Geometry check sheet. Reference: drawing and pictorial views, mm from the part's lowest x, y, z. Give positions to 0.01 mm unless a question says otherwise; leave off trailing zeros. Order: outer loops, then holes, each group sorted by start corner. A loop starts at its lowest first (then second) coordinate and runs counter-clockwise, first axis right, second up.
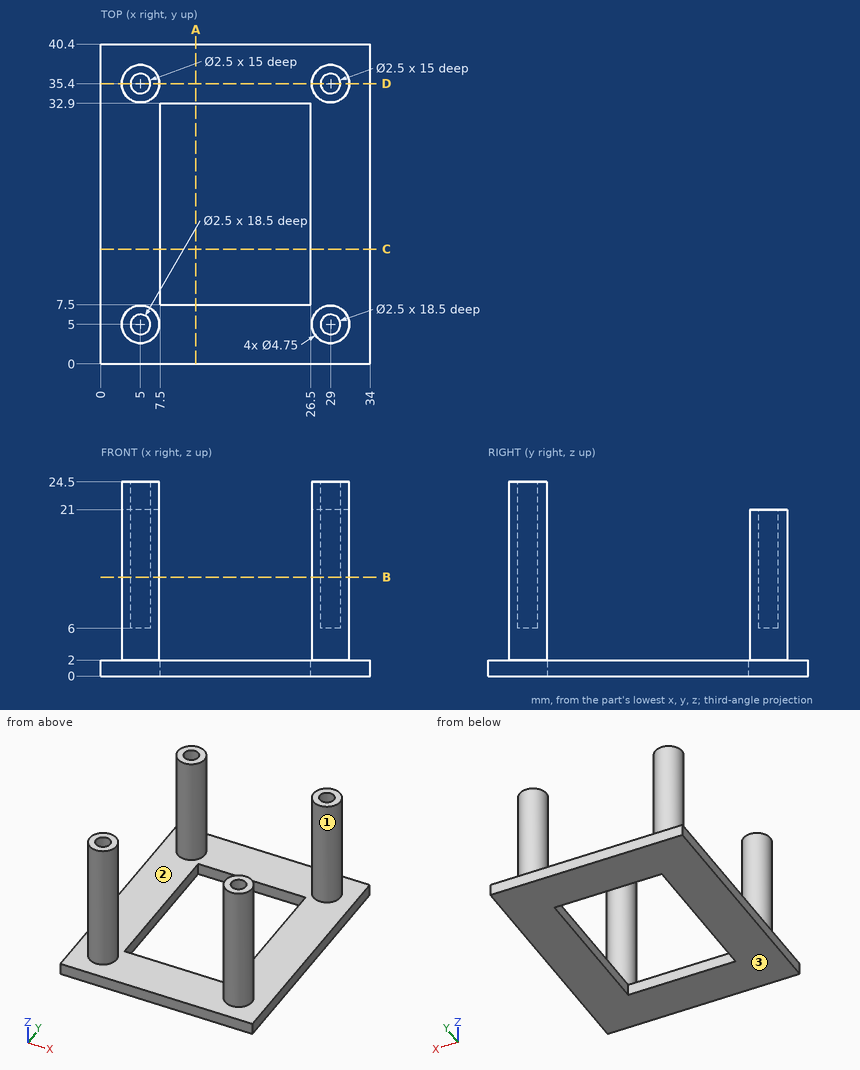
1) Depth check by flat-ended pin: pin 1 Ø1.5 at (x, y) = (5, 5) entering from +Z; pin 2 Ø4 at (x, z) = (8.5, 6.5) entering from -Y; pin 3 Ø1.6 at (x, z) = (16.5, 0.5) entering from -Y; pin 4 Ø3 at (x, y) = (4.5, 35.5) entering from +Z. Enter the tip coordinate at first touch or a pass-through.
Recorded:
pin 1: stops at z = 6
pin 2: stops at y = 3.16
pin 3: stops at y = 0
pin 4: stops at z = 21
2) Section check D-D, the plane y = 35.4. Record the cut outline in (x, z) (3 decimals).
Recorded:
outline: (0, 0) - (34, 0) - (34, 2) - (31.375, 2) - (31.375, 21) - (30.25, 21) - (30.25, 6) - (27.75, 6) - (27.75, 21) - (26.625, 21) - (26.625, 2) - (7.375, 2) - (7.375, 21) - (6.25, 21) - (6.25, 6) - (3.75, 6) - (3.75, 21) - (2.625, 21) - (2.625, 2) - (0, 2) - close
3) Material ranges on L1, parallel to Y at x = 29, z = 11.5 (3 decimals); L2, parallel to Z at x = 27, y = 25; L3, parallel to Y at x = 3, z = 3.25, recorded low to high.
Recorded:
L1: y = 2.625 to 3.75, 6.25 to 7.375, 33.025 to 34.15, 36.65 to 37.775
L2: z = 0 to 2
L3: y = 3.72 to 6.28, 34.12 to 36.68
4) Section check B-B, the plane z = 12.5. Record the cut outline in (x, y) (3 decimals), then the cut area to 3 significant figures.
Recorded:
outline: circle Ø4.75 at (5, 5); circle Ø4.75 at (5, 35.4); circle Ø4.75 at (29, 5); circle Ø4.75 at (29, 35.4); hole circle Ø2.5 at (5, 5); hole circle Ø2.5 at (5, 35.4); hole circle Ø2.5 at (29, 5); hole circle Ø2.5 at (29, 35.4)
area: 51.2 mm2
5) Draft check along Y on the marked faces 1, 2 and 3. Enter one of: +Y half, -Y half, draft (parallel to the pull), parting line (faces both ways), or undercut.
Recorded:
face 1: undercut
face 2: undercut
face 3: draft
6) Section check C-C, the plane y = 14.5. Record the cut outline in (x, z).
Recorded:
outline: (0, 0) - (7.5, 0) - (7.5, 2) - (0, 2) - close; (26.5, 0) - (34, 0) - (34, 2) - (26.5, 2) - close
7) Section check A-A, the plane x = 12. Record the cut outline in (y, z).
Recorded:
outline: (0, 0) - (7.5, 0) - (7.5, 2) - (0, 2) - close; (32.9, 0) - (40.4, 0) - (40.4, 2) - (32.9, 2) - close
